Here's the drawing with two shaded views (mm, measured from the low corner). I have some questions. Round coordinates to 2 decimals unless told otherwise and drop trailing zeros. Order: outer loops, then holes, each group sorted by start corner. A loop starts at its lowest first (then second) coordinate and runs counter-clockwise, first axis right, second up. Notation, with made-up numbers: (88, 60) -> (112, 60) arc R19 cw to (112, 71) -> close; hole circle Ø3 at (59.25, 38.25). An arc over 180 degrees is marked (long way). Answer in a Markdown table with one row per item.
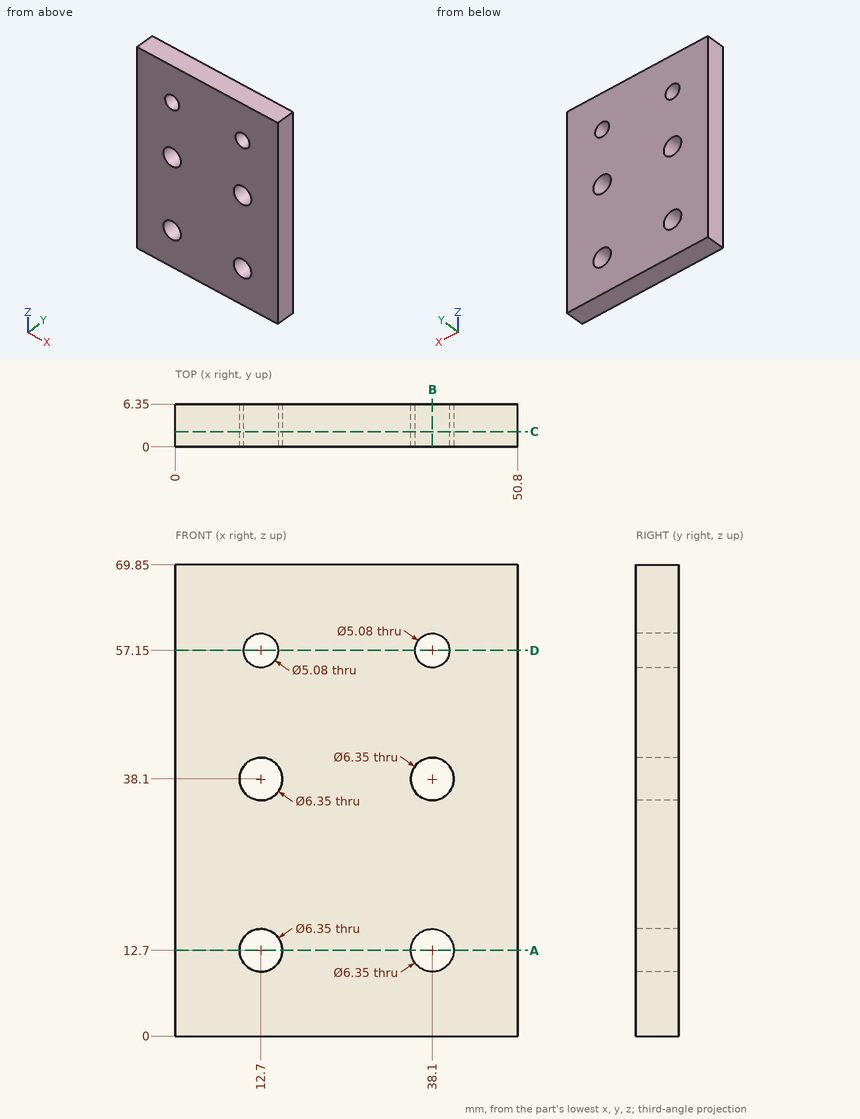
1. Suppose I cut it at A-A on z = 12.7. Write out the boundary of the cut face in (x, y) (3 decimals), then the cut area to 3 significant figures.
Numbers:
| item | result |
|---|---|
| outline | (0, 0) -> (9.525, 0) -> (9.525, 6.35) -> (0, 6.35) -> close; (15.875, 0) -> (34.925, 0) -> (34.925, 6.35) -> (15.875, 6.35) -> close; (41.275, 0) -> (50.8, 0) -> (50.8, 6.35) -> (41.275, 6.35) -> close |
| area | 242 mm2 |
2. Please list where these lines run through material, in increasing order: line 1 along Z through (x, y) = (38.1, 4.5) (3 decimals); line 2 along X through (y, z) = (2.25, 38.1) (3 decimals); line 3 along X through (y, z) = (5, 37).
Numbers:
| item | result |
|---|---|
| line 1 | z = 0 to 9.525, 15.875 to 34.925, 41.275 to 54.61, 59.69 to 69.85 |
| line 2 | x = 0 to 9.525, 15.875 to 34.925, 41.275 to 50.8 |
| line 3 | x = 0 to 9.72, 15.68 to 35.12, 41.08 to 50.8 |
3. For pin 1 Ø4 at (x, z) = (38.1, 57.15) entering from +Y, with a flat end and sliding along its axis, tell me the tip position at first contact or that it passes through.
Numbers:
| item | result |
|---|---|
| pin 1 | passes through |
4. Suppose I cut it at D-D on z = 57.15. Write out the boundary of the cut face in (x, y), then the cut area to 3 significant figures.
Numbers:
| item | result |
|---|---|
| outline | (0, 0) -> (10.16, 0) -> (10.16, 6.35) -> (0, 6.35) -> close; (15.24, 0) -> (35.56, 0) -> (35.56, 6.35) -> (15.24, 6.35) -> close; (40.64, 0) -> (50.8, 0) -> (50.8, 6.35) -> (40.64, 6.35) -> close |
| area | 258 mm2 |
5. Suppose I cut it at B-B on x = 38.1. Write out the boundary of the cut face in (y, z) (3 decimals).
Numbers:
| item | result |
|---|---|
| outline | (0, 0) -> (6.35, 0) -> (6.35, 9.525) -> (0, 9.525) -> close; (0, 15.875) -> (6.35, 15.875) -> (6.35, 34.925) -> (0, 34.925) -> close; (0, 41.275) -> (6.35, 41.275) -> (6.35, 54.61) -> (0, 54.61) -> close; (0, 59.69) -> (6.35, 59.69) -> (6.35, 69.85) -> (0, 69.85) -> close |
6. Suppose I cut it at C-C on y = 2.25. Write out the boundary of the cut face in (x, z) (3 decimals), then the cut area to 3 significant figures.
Numbers:
| item | result |
|---|---|
| outline | (0, 0) -> (50.8, 0) -> (50.8, 69.85) -> (0, 69.85) -> close; hole circle Ø6.35 at (12.7, 12.7); hole circle Ø6.35 at (12.7, 38.1); hole circle Ø5.08 at (12.7, 57.15); hole circle Ø6.35 at (38.1, 12.7); hole circle Ø6.35 at (38.1, 38.1); hole circle Ø5.08 at (38.1, 57.15) |
| area | 3,380 mm2 |
